from build123d import *

# Parameters (mm, degrees)
SKETCH_1_W              = 200
SKETCH_1_H              = 200
EXTRUDE_1_DEPTH         = 3
SKETCH_2_R              = 1.55
CUT_EXTRUDE_2_DEPTH     = 10
CUT_EXTRUDE_3_DEPTH     = 10
SKETCH_6_R              = 1.55
CUT_EXTRUDE_3_1_1_DEPTH = 10
SKETCH_7_R              = 1.55
CUT_EXTRUDE_3_1_2_DEPTH = 120.306328416
CUT_EXTRUDE_21_DEPTH    = 10


with BuildPart() as part:
    # 草图1 → 凸台-拉伸1 (new body)
    with BuildSketch(Plane(origin=(0, 0, 0), x_dir=(1, 0, 0), z_dir=(0, 1, 0))):
        Rectangle(SKETCH_1_W, SKETCH_1_H)
    extrude(amount=EXTRUDE_1_DEPTH)

    # 草图2 → 切除-拉伸2 (cut)
    with BuildSketch(Plane(origin=(0, 3, 0), x_dir=(1, 0, 0), z_dir=(0, 1, 0))):
        with Locations(Location((29.5, 9.5, 0), (0, 0, 270))):
            Circle(SKETCH_2_R)
        with Locations(Location((21.5, 0, 0), (0, 0, 270))):
            Circle(SKETCH_2_R)
        with Locations(Location((29.5, -9.5, 0), (0, 0, 270))):
            Circle(SKETCH_2_R)
        with Locations(Location((37.5, 0, 0), (0, 0, 270))):
            Circle(SKETCH_2_R)
        with Locations(Location((-29.5, -9.5, 0), (0, 0, 270))):
            Circle(SKETCH_2_R)
        with Locations(Location((-37.5, 0, 0), (0, 0, 270))):
            Circle(SKETCH_2_R)
        with Locations(Location((-21.5, 0, 0), (0, 0, 270))):
            Circle(SKETCH_2_R)
        with Locations(Location((-29.5, 9.5, 0), (0, 0, 270))):
            Circle(SKETCH_2_R)
        with Locations(Location((-15, -32, 0), (0, 0, 270))):
            Circle(SKETCH_2_R)
        with Locations(Location((15, -32, 0), (0, 0, 270))):
            Circle(SKETCH_2_R)
    extrude(amount=-CUT_EXTRUDE_2_DEPTH, mode=Mode.SUBTRACT)

    # 草图5 → 切除-拉伸3 (cut)
    with BuildSketch(Plane(origin=(0, 3, 0), x_dir=(1, 0, 0), z_dir=(0, 1, 0))):
        with BuildLine():
            Line((-65, -100), (-189.497959863, -100))
            Line((-189.497959863, -100), (-189.497959863, 163.072140164))
            Line((-189.497959863, 163.072140164), (202.300249071, 163.072140164))
            Line((202.300249071, 163.072140164), (202.300249071, -100))
            Line((202.300249071, -100), (65, -100))
            Line((65, -100), (65, -19))
            ThreePointArc((65, -19), (62.363961031, -12.636038969), (56, -10))
            Line((56, -10), (53.5, -10))
            ThreePointArc((53.5, -10), (47.136038969, -7.363961031), (44.5, -1))
            Line((44.5, -1), (44.5, 0))
            ThreePointArc((44.5, 0), (40.212142643, 10.5), (29.8, 14.9969997))
            ThreePointArc((29.8, 14.9969997), (22.858571571, 17.9949995), (20, 24.9949995))
            Line((20, 24.9949995), (20, 47.5))
            Line((20, 47.5), (0, 47.5))
            Line((0, 47.5), (-20, 47.5))
            Line((-20, 47.5), (-20, 24.9949995))
            ThreePointArc((-20, 24.9949995), (-22.858571571, 17.9949995), (-29.8, 14.9969997))
            ThreePointArc((-29.8, 14.9969997), (-40.212142643, 10.5), (-44.5, 0))
            Line((-44.5, 0), (-44.5, -1))
            ThreePointArc((-44.5, -1), (-47.136038969, -7.363961031), (-53.5, -10))
            Line((-53.5, -10), (-56, -10))
            ThreePointArc((-56, -10), (-62.363961031, -12.636038969), (-65, -19))
            Line((-65, -19), (-65, -100))
        make_face()
    extrude(amount=-CUT_EXTRUDE_3_DEPTH, mode=Mode.SUBTRACT)

    # 草图6 → φ3.1通孔1 (cut)
    with BuildSketch(Plane.XZ):
        with Locations(Location((-15, -42.5, 0), (0, 0, 270))):
            Circle(SKETCH_6_R)
        with Locations(Location((-15, -27.5, 0), (0, 0, 270))):
            Circle(SKETCH_6_R)
        with Locations(Location((15, -27.5, 0), (0, 0, 90))):
            Circle(SKETCH_6_R)
        with Locations(Location((15, -42.5, 0), (0, 0, 90))):
            Circle(SKETCH_6_R)
    extrude(amount=-CUT_EXTRUDE_3_1_1_DEPTH, mode=Mode.SUBTRACT)

    # 草图7 → φ3.1通孔2 (cut, through all)
    with BuildSketch(Plane(origin=(0, 3, 0), x_dir=(1, 0, 0), z_dir=(0, 1, 0))):
        with Locations(Location((-61, -28.5, 0), (0, 0, 270))):
            Circle(SKETCH_7_R)
        with Locations(Location((-61, -50.5, 0), (0, 0, 270))):
            Circle(SKETCH_7_R)
        with Locations(Location((61, -28.5, 0), (0, 0, 270))):
            Circle(SKETCH_7_R)
        with Locations(Location((61, -50.5, 0), (0, 0, 270))):
            Circle(SKETCH_7_R)
    extrude(amount=-CUT_EXTRUDE_3_1_2_DEPTH, mode=Mode.SUBTRACT)

    # 草图9 → φ21拨单电机孔 (cut)
    with BuildSketch(Plane(origin=(0, 3, 0), x_dir=(1, 0, 0), z_dir=(0, 1, 0))):
        with BuildLine():
            Line((-13.5, -51.75), (-13.5, -73.75))
            ThreePointArc((-13.5, -73.75), (0, -87.25), (13.5, -73.75))
            Line((13.5, -73.75), (13.5, -51.75))
            ThreePointArc((13.5, -51.75), (0, -38.25), (-13.5, -51.75))
        make_face()
    extrude(amount=-CUT_EXTRUDE_21_DEPTH, mode=Mode.SUBTRACT)


solid = part.part
Build history of the part. All positions in model axes, mm. A direction names the side the tool comes from. Coordinates: 2 decimals unless noted, no trailing zeros. Write each loop counter-clockwise with the first axis right and the second up, starting at its lowest first coordinate (ties: lowest second). Pieces come first, ordered by that corner, then holes.
(1) Mould opens along Z. For faces 1 (the cylindrical face through (-59.463, 1.521, 28.298)), 2 (the flat face through (-1, 1, 100)), 3 (the flat face through (-1, 0, 25)) say: pulls with the +Z half, pulls with the -Z half, needs draft (parallel to the pull), parting line crosses it, or undercut.
(2) Cut at B-B on z = 43. List the corners of the cut face in (x, y).
(3) Drill centre lines: line 1 (X direction, y = 1.55, z = -42.5); line 2 (X direction, y = 1, z = 28.5); line 3 (X direction, y = 2.6, z = 64.5). Where is each one in solid material? Low to high.
(4) Cut at D-D on x = 25.5. List the corners of the cut face in (y, z).
(5) Cut at C-C on y = 1.2. State how many separate pieces and enclosed holes the cut face has, and give its area (3 significant figures).
(6) Cut at A-A on x = 0. List the corners of the cut face in (y, z).
(7) 3-axis set-ups, long thin cutter, end or side, ignore diameter. For faces 4 (the flat face through (-20, 2, -36)), 5 (the flat face through (-65, 2, 59)), 6 (the cylindrical face through (0.297, 1.521, 38.253)): which of +Z, -Z, +X, -X, +Y, -Y reach the whole face in a straight line?
(8) Pin check, flat tips, straight feed: pin 1 Ø0.8 at (x, y) = (55, 2) entering from -Z; pin 2 Ø3.5 at (x, z) = (15, -42.5) entering from +Y; pin 3 Ø1.1 at (y, z) = (1, 0.5) entering from +X. Stop position of each tip, or through.
Working result:
1. face 1: undercut
1. face 2: pulls with the +Z half
1. face 3: needs draft
2. outline: (-65, 0) - (-10.28, 0) - (-10.28, 3) - (-65, 3) - close; (10.28, 0) - (65, 0) - (65, 3) - (10.28, 3) - close
3. line 1: x = -20 to -16.55, -13.45 to 13.45, 16.55 to 20
3. line 2: x = -65 to -62.55, -59.45 to 59.45, 62.55 to 65
3. line 3: x = -65 to -13.5, 13.5 to 65
4. outline: (0, -16.06) - (3, -16.06) - (3, 100) - (0, 100) - close
5. separate pieces: 1
5. enclosed holes: 19
5. area: 13,900 mm2
6. outline: (0, -47.5) - (3, -47.5) - (3, 38.25) - (0, 38.25) - close; (0, 87.25) - (3, 87.25) - (3, 100) - (0, 100) - close
7. face 4: -Z, -X, +Y, -Y
7. face 5: +Z, -Z, -X, +Y, -Y
7. face 6: +Y, -Y
8. pin 1: stops at z = 10
8. pin 2: stops at y = 3
8. pin 3: stops at x = 44.5
